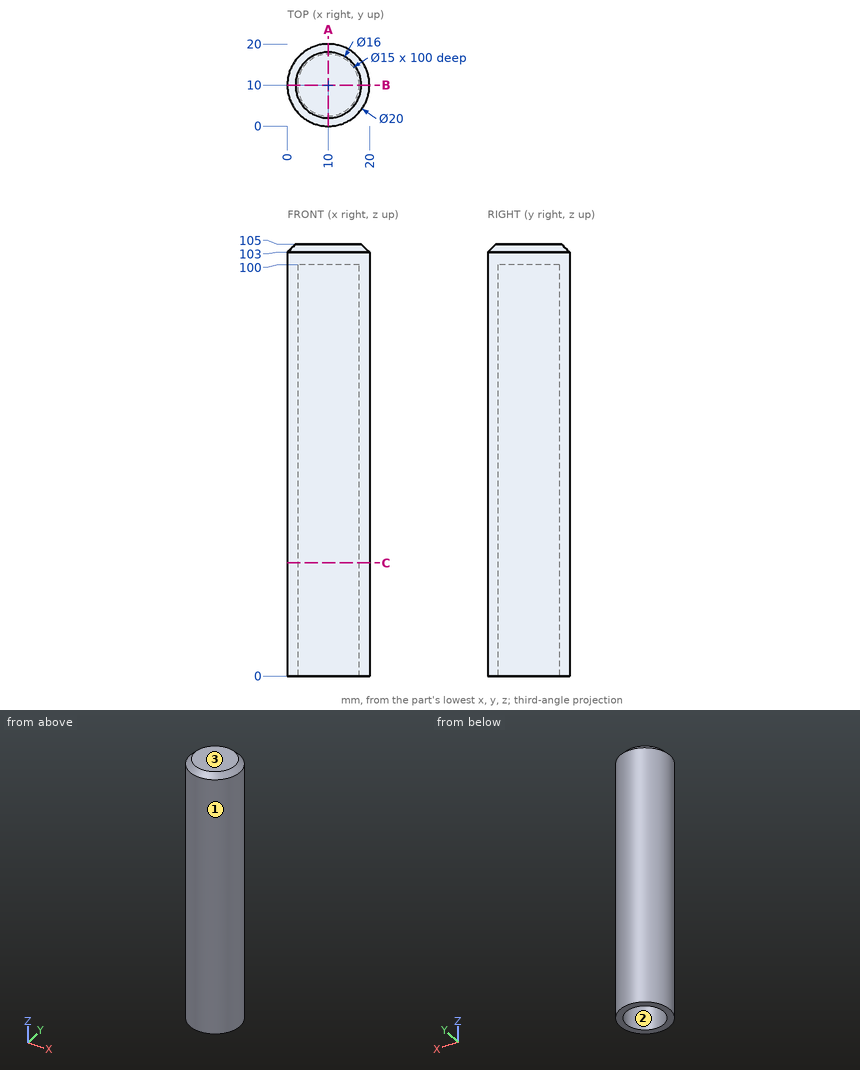
Could you check a few things on this drawing? It's one solid part, dimensions in mm from its lowest x, y, z. Coordinates: 2 decimals unless noted, no trailing zeros. Write each loop counter-clockwise with the first axis right and the second up, starting at its lowest first coordinate (ties: lowest second). Pieces come first, ordered by that corner, then holes.
Q1. Imagine slicing it at A-A, the plane x = 10. List the corners of the cut face in (y, z) for me, plus the area to 3 significant figures.
Results found:
outline: (0, 0) - (2.5, 0) - (2.5, 100) - (17.5, 100) - (17.5, 0) - (20, 0) - (20, 103) - (18, 105) - (2, 105) - (0, 103) - close
area: 596 mm2
Q2. Please list where these lines run through material, in increasing order: L1, parallel to Y at x = 10, z = 64; L2, parallel to Z at x = 4.5, y = 8.25; L3, parallel to X at y = 13, z = 52.
Results found:
L1: y = 0 to 2.5, 17.5 to 20
L2: z = 100 to 105
L3: x = 0.46 to 3.13, 16.87 to 19.54
Q3. Imagine slicing it at C-C, the plane z = 27.5. List the corners of the cut face in (x, y) for me.
Results found:
outline: circle Ø20 at (10, 10); hole circle Ø15 at (10, 10)
Q4. If we mould it in two halves opening along X, with no side actions, what happens to the marked faces 1, 2 and 3? For each: +X half, -X half, draft (parallel to the pull), parting line (faces both ways), or undercut.
Results found:
face 1: parting line
face 2: undercut
face 3: draft
Q5. For P1, Ø5, axis at y = 4, z = 60.5, coming from the -X side; P2, Ø10, axis at x = 3.5, z = 25.5, coming from the -Y side; P3, Ø1.5, axis at y = 8, z = 39.5, coming from the -X side, each with a flat end and sliding along its axis, tell me the tip position at first contact or that it passes through.
Results found:
P1: stops at x = 0.63
P2: stops at y = 0.11
P3: stops at x = 0.08
